Read the model definition and answer for the solid it produces. Units are mm, in the model's axes. A direction names the side the tool comes from. Round coordinates to 2 decimals unless told otherwise and drop trailing zeros. Order: outer loops, then holes, each group sorted by start corner. A loop starts at its lowest first (then second) coordinate and runs counter-clockwise, first axis right, second up. Notation, with made-up numbers: (-8.5, -34) - (29.5, -34) arc R14 cw to (29.5, -12) - close; hole circle Ø8 at (11, 84.25). An arc over 180 degrees is marked (long way). Put each result on its own line as item: value. Start each with the question number.
Q1. Section B-B on z = 132 is taken. Give the vertices of the cut face in (x, y), then the cut area to 3 significant figures.
Q2. For a pull along Z with two mould halves and no side action, classify faces 1 (the face through (-60.12, -46.1, 87.66)), 2 (the face through (15, -15, 101.6)), 3 (the face through (50, -50, 177.8)) as pulls with the +Z half, pulls with the -Z half, needs draft (parallel to the pull), parting line crosses it, or undercut.
Q3. Which of the six approach directions +Z, -Z, +X, -X, +Y, -Y give full straight-line access (tool end or side, diameter ignored) to faces 4 (the face through (67.266, 21.183, 140.233)), 5 (the face through (-4.347, -19.575, 155.445)), 6 (the face through (65.2, -20.5, 43.8)), 7 (the face through (-12, 68, 0)), 8 (the face through (0, 0, 228.6))?
Q4. Section A-A on y = -26 is taken. Give the vertices of the cut face in (x, z).
Q5. Section C-C on x = -31.5 is taken. Give the vertices of the cut face in (y, z), then the cut area to 3 significant figures.
Q6. Each of these flat-tipped pins is pushed along its axis until it touches: pin 1 Ø1 at (y, z) = (57.5, 179.5) entering from +X; pin 2 Ø12 at (y, z) = (25, 97) entering from +X; pin 3 Ø3 at (x, y) = (-41, 57) entering from +Z; pin 4 Ø8 at (x, z) = (57, 56.5) entering from -Y. Where does it stop, or does it pass through?
Q7. Section D-D on x = 0 is taken. Give the vertices of the cut face in (y, z), then the cut area to 3 significant figures.
Q8. Find the intervals of material crossed by line 1 along Y through (x, z) = (0, 152.5); line 2 along Y through (x, z) = (0, 37); line 3 along Z through (x, y) = (-38, 49), in increasing order. Write a range as from..to.
from build123d import *

# Parameters (mm, degrees)
F0_R     = 75.759685
F1_DEPTH = 177.8
F2_R     = 70.52244
F3_DEPTH = 76.2
F4_R     = 20.051342
F5_DEPTH = 127
F6_R     = 35.247261
F6_R_2   = 20.051342
F7_DEPTH = 17.78
F8_R     = 68.34828
F9_DEPTH = 88.9


with BuildPart() as f1:
    # F0 (on Top) → F1 (new body)
    with BuildSketch(Plane.XY):
        Circle(F0_R)
    extrude(amount=F1_DEPTH)

    # F2 (on face) → F3 (cut)
    with BuildSketch(Plane.XY.offset(177.8)):
        Circle(F2_R)
    extrude(amount=-F3_DEPTH, mode=Mode.SUBTRACT)

    # F4 (on face) → F5 (join)
    with BuildSketch(Plane.XY.offset(101.6)):
        Circle(F4_R)
    extrude(amount=F5_DEPTH)

    # F6 (on face) → F7 (join)
    with BuildSketch(Plane.XY.offset(228.6)):
        Circle(F6_R)
        Circle(F6_R_2, mode=Mode.SUBTRACT)
    extrude(amount=-F7_DEPTH)

    # F8 (on face) → F9 (cut)
    with BuildSketch(Plane(origin=(0, 0, 0), x_dir=(1, 0, 0), z_dir=(0, 0, -1))):
        Circle(F8_R)
    extrude(amount=-F9_DEPTH, mode=Mode.SUBTRACT)


solid = f1.part
Findings:
1. outline: circle Ø151.52 at (0, 0); circle Ø40.1 at (0, 0); hole circle Ø141.04 at (0, 0)
1. area: 3,670 mm2
2. face 1: needs draft
2. face 2: undercut
2. face 3: pulls with the +Z half
3. face 4: +Z
3. face 5: none
3. face 6: -Z
3. face 7: -Z, +X, -X, +Y, -Y
3. face 8: +Z, +X, -X, +Y, -Y
4. outline: (-71.16, 0) - (-63.21, 0) - (-63.21, 88.9) - (63.21, 88.9) - (63.21, 0) - (71.16, 0) - (71.16, 177.8) - (65.55, 177.8) - (65.55, 101.6) - (-65.55, 101.6) - (-65.55, 177.8) - (-71.16, 177.8) - close; (-23.8, 210.82) - (23.8, 210.82) - (23.8, 228.6) - (-23.8, 228.6) - close
5. outline: (-68.9, 0) - (-60.66, 0) - (-60.66, 88.9) - (60.66, 88.9) - (60.66, 0) - (68.9, 0) - (68.9, 177.8) - (63.1, 177.8) - (63.1, 101.6) - (-63.1, 101.6) - (-63.1, 177.8) - (-68.9, 177.8) - close; (-15.82, 210.82) - (15.82, 210.82) - (15.82, 228.6) - (-15.82, 228.6) - close
5. area: 4,660 mm2
6. pin 1: through
6. pin 2: x = 73.34
6. pin 3: z = 177.8
6. pin 4: y = -54.13
7. outline: (-75.76, 0) - (-68.35, 0) - (-68.35, 88.9) - (68.35, 88.9) - (68.35, 0) - (75.76, 0) - (75.76, 177.8) - (70.52, 177.8) - (70.52, 101.6) - (20.05, 101.6) - (20.05, 210.82) - (35.25, 210.82) - (35.25, 228.6) - (-35.25, 228.6) - (-35.25, 210.82) - (-20.05, 210.82) - (-20.05, 101.6) - (-70.52, 101.6) - (-70.52, 177.8) - (-75.76, 177.8) - close
7. area: 9,670 mm2
8. line 1: -75.76..-70.52, -20.05..20.05, 70.52..75.76
8. line 2: -75.76..-68.35, 68.35..75.76
8. line 3: 88.9..101.6
